Verification items for this drawing (mm, ordinates from the low corner). Give positions to 0.01 mm unless a question says otherwise; leave off trailing zeros. Write each loop counter-clockwise with the first axis right and the second up, starting at its lowest first coordinate (ties: lowest second). Pieces come first, ordered by that corner, then holes. Notation, with made-up numbers: (45.5, 43.25) -> (84.5, 43.25) arc R20 cw to (84.5, 53.25) -> close; hole circle Ø1 at (64, 17.25). An arc over 180 degrees is marked (long way). Use one line per item in the form item = value. Start each with the question number.
(1) Scan lines: L1, parallel to X at y = 3.8, z = 12; L2, parallel to Z at x = 37.5, y = 3.1; L3, parallel to Z at x = 233.5, y = 1.5. Record each from-to range of solid material in increasing order.
(2) Section check A-A, the plane y = 2. Record the cut outline in (x, z), plus the area to 3 significant figures.
(3) Section check B-B, the plane x = 57. Record the cut outline in (y, z), plus the area to 3 significant figures.
(4) Depth check by flat-ended pin: pin 1 Ø5 at (x, z) = (233.5, 12) entering from +Y; pin 2 Ø6 at (x, z) = (134, 6) entering from +Y; pin 3 Ø4 at (x, z) = (55, 18) entering from +Y. Enter the tip coordinate at first touch or a pass-through.
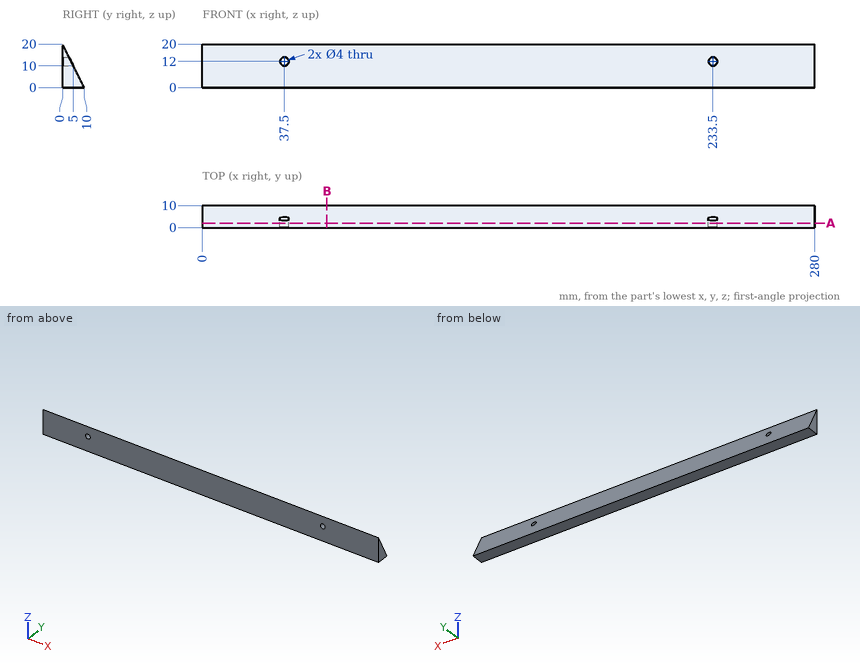
Completed:
q1.L1 = 0 to 35.5, 39.5 to 231.5, 235.5 to 280
q1.L2 = 0 to 10
q1.L3 = 0 to 10, 14 to 17
q2.outline = (0, 0) -> (280, 0) -> (280, 16) -> (0, 16) -> close; hole circle Ø4 at (37.5, 12); hole circle Ø4 at (233.5, 12)
q2.area = 4,450 mm²
q3.outline = (0, 0) -> (10, 0) -> (0, 20) -> close
q3.area = 100 mm²
q4.pin_1 = 5.25
q4.pin_2 = 8.5
q4.pin_3 = 2
